from build123d import *

# Parameters (mm, degrees)
F3_D = 3.7973
F6_D = 2.7051
F7_R = 0.762


with BuildPart() as f1:
    # F0 (on Right) → F1 (revolve)
    with BuildSketch(Plane.YZ):
        Polygon((0, 15.875), (-31.75, 15.875), (-31.75, 9.525), (-6.35, 9.525), (-6.35, 0), (15.1730990037, 0), (15.1730990037, 6.35), align=None)
    revolve(axis=Axis((0, 4.4115495019, 0), (0, 1, 0)))

    # F3 (through all)
    with Locations(Plane(origin=(0, 15.1730990037, 0), x_dir=(-1, 0, 0), z_dir=(0, 1, 0))):
        with Locations((0, 0)):
            Hole(F3_D / 2)

    # F6 (through all)
    with Locations(Plane.XY.offset(17.018)):
        with Locations((0, -19.05)):
            Hole(F6_D / 2)

    # F7
    f7_edges = [f1.edges().sort_by_distance(p)[0] for p in [
        (0, 15.173099, -6.35),
        (0, 0, -15.875),
    ]]
    fillet(f7_edges, radius=F7_R)


solid = f1.part
Check sheet for the modelled part. Datum: model origin and axes. Units: mm. A direction names the side the tool comes from. Round coordinates to 2 decimals unless told otherwise and drop trailing zeros. Write each loop counter-clockwise with the first axis right and the second up, starting at its lowest first coordinate (ties: lowest second). Pieces come first, ordered by that corner, then holes. Notation, with made-up numbers: (-22.75, 19) - (19.25, 19) arc R13 ccw to (19.25, 34) - close; hole circle Ø4 at (59.5, -24). An arc over 180 degrees is marked (long way). Return JSON: item names as keys, results as strings.
Q1. Access from +Z, -Z, +X, -X, +Y, -Y to the whole of each face (thin tool, end or side, straight path). Record for faces 1 (the cylindrical face through (2.861, -18.872, 9.085)), 2 (the cylindrical face through (-0.62, -20.25, 12.61)).
Returned:
{"face 1": "-Y", "face 2": "+Z, -Z"}
Q2. Depth check by flat-ended pin: P1, Ø15, axis at x = 0, z = 1, coming from the -Y side; P2, Ø12, axis at x = 9.5, y = -14.5, coming from the -Z side; P3, Ø2, axis at x = 4, y = -20.5, coming from the -Z side. Enter the tip coordinate at first touch or a pass-through.
Returned:
{"P1": "stops at y = -6.35", "P2": "stops at z = -15.48", "P3": "stops at z = -15.59"}
Q3. Cross-section at C-C (y = -19.05). Record the boundary of the cut face in (x, z) (3 decimals).
Returned:
{"outline": "(-1.353, -15.817) - (-1.353, -9.428) arc R9.525 cw to (-1.353, 9.428) - (-1.353, 15.817) arc R15.875 ccw to start; (1.353, -15.817) arc R15.875 ccw to (1.353, 15.817) - (1.353, 9.428) arc R9.525 cw to (1.353, -9.428) - close"}
Q4. Cross-section at B-B (x = 0). Give the number of separate pieces and of enclosed holes in the cut face, then the cut area to 3 significant figures.
Returned:
{"separate pieces": "4", "enclosed holes": "0", "area": "745 mm²"}
Q5. Cross-section at A-A (y = -24). Record the boundary of the cut face in (x, z) (3 decimals).
Returned:
{"outline": "circle Ø31.75 at (0, 0); hole circle Ø19.05 at (0, 0)"}
Q6. Draft check along Z on faces 3 (the cylindrical face through (-6.08, -16.205, 14.664)), 4 (the cylindrical face through (1.8, 4.3, 0.6)), 5 (the flat face through (-7, -31.75, 7)). Enter one of: released by +Z, released by -Z, zero draft, split by the parting line, or undercut.
Returned:
{"face 3": "split by the parting line", "face 4": "undercut", "face 5": "zero draft"}
Q7. Scan lines: L1, parallel to Z at x = 0, y = -24 (3 decimals); L2, parallel to Z at x = 0, y = 3.5; L3, parallel to Y at x = 0, z = 12. Record each from-to range of solid material in increasing order. Write a range as from..to.
Returned:
{"L1": "z = -15.875..-9.525, 9.525..15.875", "L2": "z = -13.68..-1.9, 1.9..13.68", "L3": "y = -31.75..-20.4, -17.7..6.17"}
